Build history of the part. All positions in model axes, mm. Face numbers are marked on the shaded views. A direction names the side the tool comes from. Give positions to 0.01 mm unless a question says otherwise; leave off trailing zeros. Loops run counter-clockwise (first coordinate to the right, second up) from the corner with the lowest first, then second, coordinate; pieces in that order, holes last.
1) 3-axis set-ups, long thin cutter, end or side, ignore diameter. For the marked faces 1, 2 and 3: which of +Z, -Z, +X, -X, +Y, -Y reach the whole face in a straight line?
2) Band-saw the part on B-B on y = -0.2. List the corners of the cut face in (x, z).
3) Flat gauge pin, fed straight in: P1, Ø0.9, axis at y = 0.5, z = 6, coming from the +X side. Where does the tip first touch, or does it go through?
4) Two-plate mould, pull along Z, no slides. Class the marked faces 4, 5, 6 and 7: +Z half, -Z half, draft (parallel to the pull), parting line (faces both ways), or undercut.
5) Band-saw the part on D-D on z = 8.5. List the corners of the cut face in (x, y), then the cut area to 3 significant figures.
6) Band-saw the part on C-C on z = 6.75. List the corners of the cut face in (x, y), then the cut area to 3 significant figures.
7) Band-saw the part on A-A on x = -3.25. List the corners of the cut face in (y, z).
8) Wall check: line 1 (Z direction, x = 4, y = 0.1); line 2 (X direction, y = 1, z = 3.25); line 3 (X direction, y = -1.2, z = 8.75). Give the ranges that are in metal, low to high.
```python
from build123d import *

# Parameters (mm, degrees)
F0_W     = 15
F0_H     = 3
F1_DEPTH = 1
F2_W     = 3
F2_H     = 3
F3_DEPTH = 10
F4_W     = 3
F4_H     = 3
F5_DEPTH = 10


with BuildPart() as f1:
    # F0 (on Top) → F1 (new body)
    with BuildSketch(Plane.XY):
        Rectangle(F0_W, F0_H)
    extrude(amount=F1_DEPTH)

    # F2 (on face) → F3 (join)
    with BuildSketch(Plane.XY.offset(1)):
        with Locations((-6, 0)):
            Rectangle(F2_W, F2_H)
    extrude(amount=F3_DEPTH)

    # F4 (on face) → F5 (join)
    with BuildSketch(Plane.YZ.offset(-4.5)):
        with Locations((0, 9.5)):
            Rectangle(F4_W, F4_H)
    extrude(amount=F5_DEPTH)


solid = f1.part
```
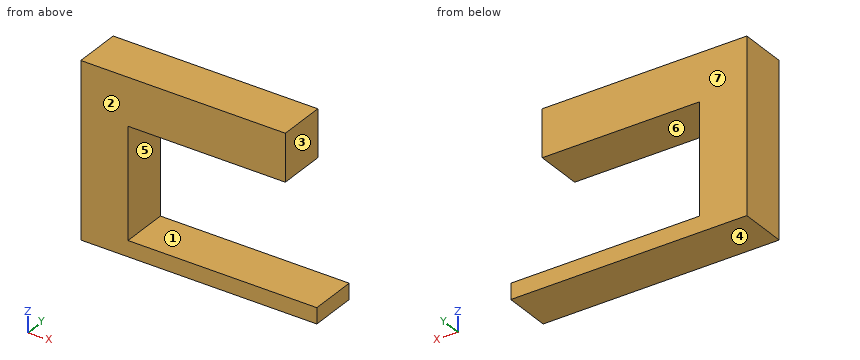
Findings below:
1. face 1: +X, +Y, -Y
1. face 2: +Z, -Z, +X, -X, -Y
1. face 3: +Z, +X, +Y, -Y
2. outline: (-7.5, 0) - (7.5, 0) - (7.5, 1) - (-4.5, 1) - (-4.5, 8) - (5.5, 8) - (5.5, 11) - (-7.5, 11) - close
3. P1: stops at x = -4.5
4. face 4: -Z half
4. face 5: undercut
4. face 6: undercut
4. face 7: draft
5. outline: (-7.5, -1.5) - (5.5, -1.5) - (5.5, 1.5) - (-7.5, 1.5) - close
5. area: 39.0 mm2
6. outline: (-7.5, -1.5) - (-4.5, -1.5) - (-4.5, 1.5) - (-7.5, 1.5) - close
6. area: 9.00 mm2
7. outline: (-1.5, 0) - (1.5, 0) - (1.5, 1) - (-1.5, 1) - close; (-1.5, 8) - (1.5, 8) - (1.5, 11) - (-1.5, 11) - close
8. line 1: z = 0 to 1, 8 to 11
8. line 2: x = -7.5 to -4.5
8. line 3: x = -7.5 to 5.5
